For this review, take the finished solid that the model builds, in its own axes (mm). Face numbers are marked on the shaded views. A direction names the side the tool comes from. Round coordinates to 2 decimals unless told otherwise and drop trailing zeros. Write each loop counter-clockwise with the first axis right and the second up, starting at its lowest first coordinate (ties: lowest second). Pieces come first, ordered by that corner, then holes. Notation, with made-up numbers: (1, 83.25) -> (26, 83.25) arc R18 cw to (26, 91.25) -> close; hole circle Ø5 at (83.25, 10.25). An arc over 180 degrees is marked (long way). Answer in a Markdown table with one row per item.
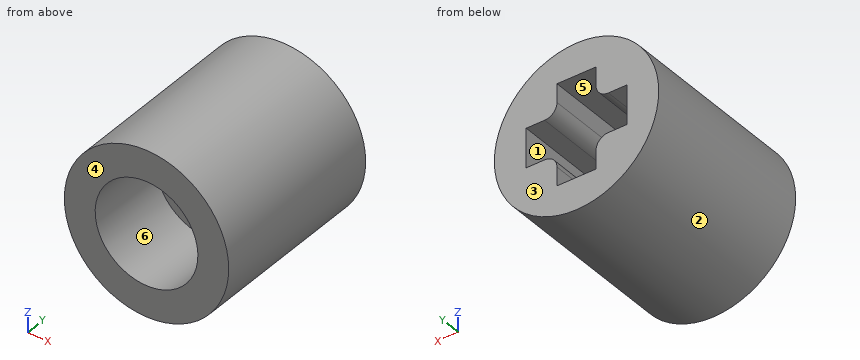
from build123d import *

# Parameters (mm, degrees)
SKETCH1_R           = 4
SKETCH1_R_2         = 2.5
BOSS_EXTRUDE1_DEPTH = 4
SKETCH3_R           = 4
BOSS_EXTRUDE2_DEPTH = 5
SKETCH4_W           = 1.5
SKETCH4_H           = 1.9
SKETCH4_W_2         = 1.9
SKETCH4_H_2         = 1.5
CUT_EXTRUDE1_DEPTH  = 4
FILLET1_R           = 0.6


with BuildPart() as part:
    # Sketch1 → Boss-Extrude1 (new body)
    with BuildSketch(Plane(origin=(0, 0, 0), x_dir=(1, 0, 0), z_dir=(0, 1, 0))):
        with Locations(Location((0, 0, 0), (0, 0, 270))):
            Circle(SKETCH1_R)
        with Locations(Location((0, 0, 0), (0, 0, 270))):
            Circle(SKETCH1_R_2, mode=Mode.SUBTRACT)
    extrude(amount=BOSS_EXTRUDE1_DEPTH)

    # Sketch3 → Boss-Extrude2 (add)
    with BuildSketch(Plane(origin=(0, 4, 0), x_dir=(1, 0, 0), z_dir=(0, 1, 0))):
        with Locations(Location((0, 0, 0), (0, 0, 270))):
            Circle(SKETCH3_R)
    extrude(amount=BOSS_EXTRUDE2_DEPTH)

    # Sketch4 → Cut-Extrude1 (cut)
    with BuildSketch(Plane(origin=(0, 9, 0), x_dir=(1, 0, 0), z_dir=(0, 1, 0))):
        with Locations((-1.7, 0)):
            Rectangle(SKETCH4_W, SKETCH4_H)
        with Locations((0, 1.7)):
            Rectangle(SKETCH4_W_2, SKETCH4_H_2)
        with Locations((1.7, 0)):
            Rectangle(SKETCH4_W, SKETCH4_H)
        Rectangle(SKETCH4_W_2, SKETCH4_H)
        with Locations((0, -1.7)):
            Rectangle(SKETCH4_W_2, SKETCH4_H_2)
    extrude(amount=-CUT_EXTRUDE1_DEPTH, mode=Mode.SUBTRACT)

    # Fillet1
    fillet1_edges = [part.edges().sort_by_distance(p)[0] for p in [
        (-0.95, 7, -0.95),
        (0.95, 7, -0.95),
        (0.95, 7, 0.95),
        (-0.95, 7, 0.95),
    ]]
    fillet(fillet1_edges, radius=FILLET1_R)


solid = part.part
1) Consider section B-B on y = 7.75. State the section outline as (x, z) points.
Solved:
| item | result |
|---|---|
| outline | circle Ø8 at (0, 0); hole (-2.45, -0.95) -> (-1.55, -0.95) arc R0.6 cw to (-0.95, -1.55) -> (-0.95, -2.45) -> (0.95, -2.45) -> (0.95, -1.55) arc R0.6 cw to (1.55, -0.95) -> (2.45, -0.95) -> (2.45, 0.95) -> (1.55, 0.95) arc R0.6 cw to (0.95, 1.55) -> (0.95, 2.45) -> (-0.95, 2.45) -> (-0.95, 1.55) arc R0.6 cw to (-1.55, 0.95) -> (-2.45, 0.95) -> close |
2) For line 1 (X direction, y = 2.1, z = 0); line 2 (X direction, y = 7.75, z = -1.75); line 3 (Y direction, x = -1.25, z = -1.5), list the stretches that pass through material, from the lowest coordinate up. Write a range as [from, to].
Solved:
| item | result |
|---|---|
| line 1 | [-4, -2.5], [2.5, 4] |
| line 2 | [-3.6, -0.95], [0.95, 3.6] |
| line 3 | [4, 9] |
3) Consider section C-C on z = -2.25. State the section outline as (x, y) points, then the cut area to 3 significant figures.
Solved:
| item | result |
|---|---|
| outline | (-3.31, 0) -> (-1.09, 0) -> (-1.09, 4) -> (1.09, 4) -> (1.09, 0) -> (3.31, 0) -> (3.31, 9) -> (0.95, 9) -> (0.95, 5) -> (-0.95, 5) -> (-0.95, 9) -> (-3.31, 9) -> close |
| area | 43.2 mm² |
4) Consider section A-A on x = 0. State the section outline as (y, z) points, then the cut area to 3 significant figures.
Solved:
| item | result |
|---|---|
| outline | (0, -4) -> (9, -4) -> (9, -2.45) -> (5, -2.45) -> (5, 2.45) -> (9, 2.45) -> (9, 4) -> (0, 4) -> (0, 2.5) -> (4, 2.5) -> (4, -2.5) -> (0, -2.5) -> close |
| area | 32.4 mm² |
5) Clearance check with flat-ended pins moving along their axes: pin 1 Ø1 at (y, z) = (6.5, 0.5) entering from +X; pin 2 Ø1 at (x, y) = (-2, 8) entering from +Z; pin 3 Ø1.5 at (x, y) = (1, 5.5) entering from -Z; pin 4 Ø0.7 at (x, y) = (-2, 8) entering from -Z. State where each tip first meets the part, or that it passes through.
Solved:
| item | result |
|---|---|
| pin 1 | x = 4 |
| pin 2 | z = 3.71 |
| pin 3 | z = -3.99 |
| pin 4 | z = -3.64 |
6) For the marked faces 4, 5 and 6, list the 3-axis set-ups (+Z, -Z, +X, -X, +Y, -Y) from which the entire face can be reached by the end or side of a thin tool; tool diameter is ignored.
Solved:
| item | result |
|---|---|
| face 4 | +Z, -Z, +X, -X, -Y |
| face 5 | +Y |
| face 6 | -Y |
7) Consider section D-D on y = 4.25. State the section outline as (x, z) points, then the cut area to 3 significant figures.
Solved:
| item | result |
|---|---|
| outline | circle Ø8 at (0, 0) |
| area | 50.3 mm² |
8) Mouldability with a two-part tool opening along Z and no side actions: class the marked faces 1, 2 and 3 as pulls with the +Z half, pulls with the -Z half, needs draft (parallel to the pull), parting line crosses it, or undercut.
Solved:
| item | result |
|---|---|
| face 1 | undercut |
| face 2 | parting line crosses it |
| face 3 | needs draft |
